Source: three-view drawing plus pictorial views. Frame: mm from the lowest corner of the part. A direction names the side the tool comes from. Give positions to 0.01 mm unless a question says otherwise; leave off trailing zeros. Loops run counter-clockwise (first coordinate to the right, second up) from the corner with the lowest first, then second, coordinate; pieces in that order, holes last. Notation, with made-up numbers: (41, 37) -> (90, 37) arc R7 ccw to (90, 41) -> close; hole circle Ø6 at (80, 47). An arc over 180 degrees is marked (long way). Put each result on its own line as item: value.
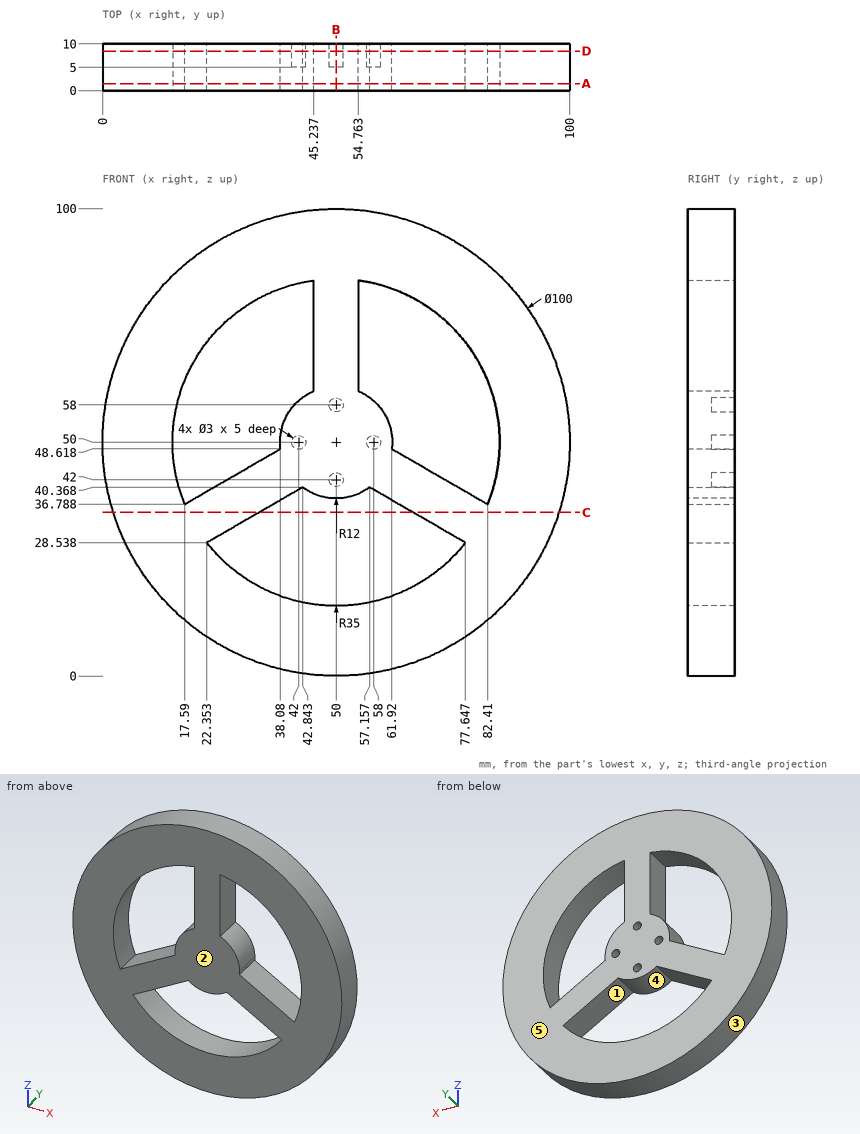
(1) Section B-B on x = 50. Return loops of the section in (y, z), then the cut area to 3 significant figures.
Calculated:
outline: (0, 0) -> (10, 0) -> (10, 15) -> (0, 15) -> close; (0, 38) -> (10, 38) -> (10, 40.5) -> (5, 40.5) -> (5, 43.5) -> (10, 43.5) -> (10, 56.5) -> (5, 56.5) -> (5, 59.5) -> (10, 59.5) -> (10, 100) -> (0, 100) -> close
area: 740 mm²
(2) Section C-C on z = 35. Return loops of the section in (x, y) (1 decimal).
Calculated:
outline: (2.3, 0) -> (33.5, 0) -> (33.5, 10) -> (2.3, 10) -> close; (66.5, 0) -> (97.7, 0) -> (97.7, 10) -> (66.5, 10) -> close
(3) First-contact query: P1, Ø3, axis at x = 79, y = 5, coming from the -Z side; P2, Ø2.5, axis at x = 50, z = 58, coming from the +Y side; P3, Ø3, axis at y = 3, z = 73.5, coming from the -X side; P4, Ø1, axis at x = 28, z = 29.5, coming from the +Y side. Flat tips, straight axial feed; report the tip coordinate or a pass-through.
Calculated:
P1: stops at z = 8.24
P2: stops at y = 5
P3: stops at x = 5.1
P4: passes through
(4) Draft query along X for the marked faces 3, 4 and 5. Return one class per face: released by +X, released by -X, zero draft, split by the parting line, or undercut.
Calculated:
face 3: split by the parting line
face 4: undercut
face 5: zero draft
(5) Section A-A on y = 1.5. Return loops of the section in (x, z) (1 decimal), then the cut area to 3 significant figures.
Calculated:
outline: circle Ø100 at (50, 50); hole (17.6, 36.8) -> (38.1, 48.6) arc R12 cw to (45.2, 61) -> (45.2, 84.7) arc R35 ccw to start; hole (22.4, 28.5) arc R35 ccw to (77.6, 28.5) -> (57.2, 40.4) arc R12 cw to (42.8, 40.4) -> close; hole (54.8, 61) arc R12 cw to (61.9, 48.6) -> (82.4, 36.8) arc R35 ccw to (54.8, 84.7) -> close
area: 5,120 mm²
(6) Line query: probe 1 along X at (y, z) = (8.25, 50); probe 2 along X at (y, z) = (6.1, 42) (1 decimal); probe 3 along X at (y, z) = (9.25, 68) (1 decimal). Output: solid intervals per line, ascending. Write a range as from..to.
Calculated:
probe 1: x = 0..15, 38..40.5, 43.5..56.5, 59.5..62, 85..100
probe 2: x = 0.6..15.9, 26.6..48.5, 51.5..73.4, 84.1..99.4
probe 3: x = 3.4..20, 45.2..54.8, 80..96.6
(7) Section D-D on y = 8.5. Return loops of the section in (x, z) (1 decimal), then the cut area to 3 significant figures.
Calculated:
outline: circle Ø100 at (50, 50); hole (17.6, 36.8) -> (38.1, 48.6) arc R12 cw to (45.2, 61) -> (45.2, 84.7) arc R35 ccw to start; hole (22.4, 28.5) arc R35 ccw to (77.6, 28.5) -> (57.2, 40.4) arc R12 cw to (42.8, 40.4) -> close; hole circle Ø3 at (42, 50); hole circle Ø3 at (50, 42); hole circle Ø3 at (50, 58); hole (54.8, 61) arc R12 cw to (61.9, 48.6) -> (82.4, 36.8) arc R35 ccw to (54.8, 84.7) -> close; hole circle Ø3 at (58, 50)
area: 5,090 mm²
(8) Reachability of the marked faces 1 and 2 from +Z, -Z, +X, -X, +Y, -Y: full face, straight path, thin tool, end or side. Return the list, or none.
Calculated:
face 1: +Y, -Y
face 2: +Z, -Z, +X, -X, -Y
